Autodesk Inventor part; units mm, degrees
ref_plane "YZ Plane" through (0, 0, 0) normal (1, 0, 0) x (0, 1, 0)
ref_plane "XZ Plane" through (0, 0, 0) normal (0, 1, 0) x (-1, 0, 0)
ref_plane "XY Plane" through (0, 0, 0) normal (0, 0, 1) x (1, 0, 0)
sketch "Sketch1" plane through (0, 0, 0) normal (0, 0, 1) x (1, 0, 0)
  circle A0 centre (0, 0) radius 10
  circle A1 centre (-6, 6) radius 1
  circle A2 centre (0, 6) radius 1
  circle A3 centre (6, 6) radius 1
  circle A4 centre (6, -6) radius 1
  circle A5 centre (0, -6) radius 1
  circle A6 centre (-6, -6) radius 1
  dimension "d0" = 20
  dimension "d2" = 2
  dimension "d3" = 12
  dimension "d4" = 6
  dimension "d5" = 12
  dimension "d6" = 6
  dimension "d7" = 6
  dimension "d8" = 2
extrude "Extrusion1" add sketch "Sketch1" along normal blind 18
sketch "Sketch2" plane through (0, 0, 18) normal (0, 0, -1) x (-1, 0, 0)
  circle A0 centre (4, 0) radius 5
  circle A1 centre (0, 6) radius 1
  point P0 (0, 0)
  dimension "d11" = 10
  dimension "d12" = 4
extrude "Extrusion2" cut sketch "Sketch2" along normal blind 18 contours A0
properties part number "11"
Source: CAD feature listing. Evaluate the final solid. Frame: model axes, mm. Round coordinates to 2 decimals unless told otherwise and drop trailing zeros. Loops run counter-clockwise (first coordinate to the right, second up) from the corner with the lowest first, then second, coordinate; pieces in that order, holes last. Notation, with made-up numbers: (53, 67) - (91, 67) arc R30 cw to (91, 97) - close; hole circle Ø2 at (67.5, 21.5). An arc over 180 degrees is marked (long way). Write item = value, one per line. Start each with the question number.
Item 1: Section query D-D on x = 6. Output: boundary loops of the cut face in (y, z), plus the area to 3 significant figures.
Item 2: First-contact query: pin 1 Ø10 at (y, z) = (-4.5, 6) entering from +X; pin 2 Ø2 at (x, z) = (7, 14) entering from +Y; pin 3 Ø1 at (y, z) = (-6, 12) entering from -X; pin 4 Ø2 at (x, z) = (2.5, 10.5) entering from -Y. Flat tips, straight axial feed; report the tip coordinate or a pass-through.
Item 3: Section query A-A on x = -8. Output: boundary loops of the cut face in (y, z).
Item 4: Mould query, pull axis X, two halves, no side actions, for faces 1 (the face through (5.263, 5.324, 8.874)), 2 (the face through (2, 0, 18)), 3 (the face through (5.263, -6.676, 8.874)), 4 (the face through (-2.17, 9.76, 8.87)). Classes: released by +X, released by -X, zero draft, split by the parting line, or undercut.
Item 5: Section query C-C on z = 1.5. Output: boundary loops of the cut face in (x, y).
Item 6: Section query B-B on y = 6. Output: boundary loops of the cut face in (x, z).
Item 7: Material intervals for line 1 (X direction, y = 0.25, z = 1.5); line 2 (X direction, y = -5.5, z = 13.75); line 3 (Y direction, x = 0, z = 10.5), sorted ascending.
Results list:
q1.outline = (-8, 0) - (-7, 0) - (-7, 18) - (-8, 18) - close; (-5, 0) - (5, 0) - (5, 18) - (-5, 18) - close; (7, 0) - (8, 0) - (8, 18) - (7, 18) - close
q1.area = 216 mm²
q2.pin_1 = 10
q2.pin_2 = 8
q2.pin_3 = -8.35
q2.pin_4 = -9.89
q3.outline = (-6, 0) - (-3, 0) - (-3, 18) - (-6, 18) - close; (3, 0) - (6, 0) - (6, 18) - (3, 18) - close
q4.face_1 = undercut
q4.face_2 = zero draft
q4.face_3 = undercut
q4.face_4 = split by the parting line
q5.outline = circle Ø20 at (0, 0); hole circle Ø10 at (-4, 0); hole circle Ø2 at (-6, -6); hole circle Ø2 at (-6, 6); hole circle Ø2 at (0, -6); hole circle Ø2 at (0, 6); hole circle Ø2 at (6, -6); hole circle Ø2 at (6, 6)
q6.outline = (-8, 0) - (-7, 0) - (-7, 18) - (-8, 18) - close; (-5, 0) - (-1, 0) - (-1, 18) - (-5, 18) - close; (1, 0) - (5, 0) - (5, 18) - (1, 18) - close; (7, 0) - (8, 0) - (8, 18) - (7, 18) - close
q7.line_1 = -10 to -8.99, 0.99 to 10
q7.line_2 = -8.35 to -6.87, -5.13 to -0.87, 0.87 to 5.13, 6.87 to 8.35
q7.line_3 = -10 to -7, -5 to -3, 3 to 5, 7 to 10
